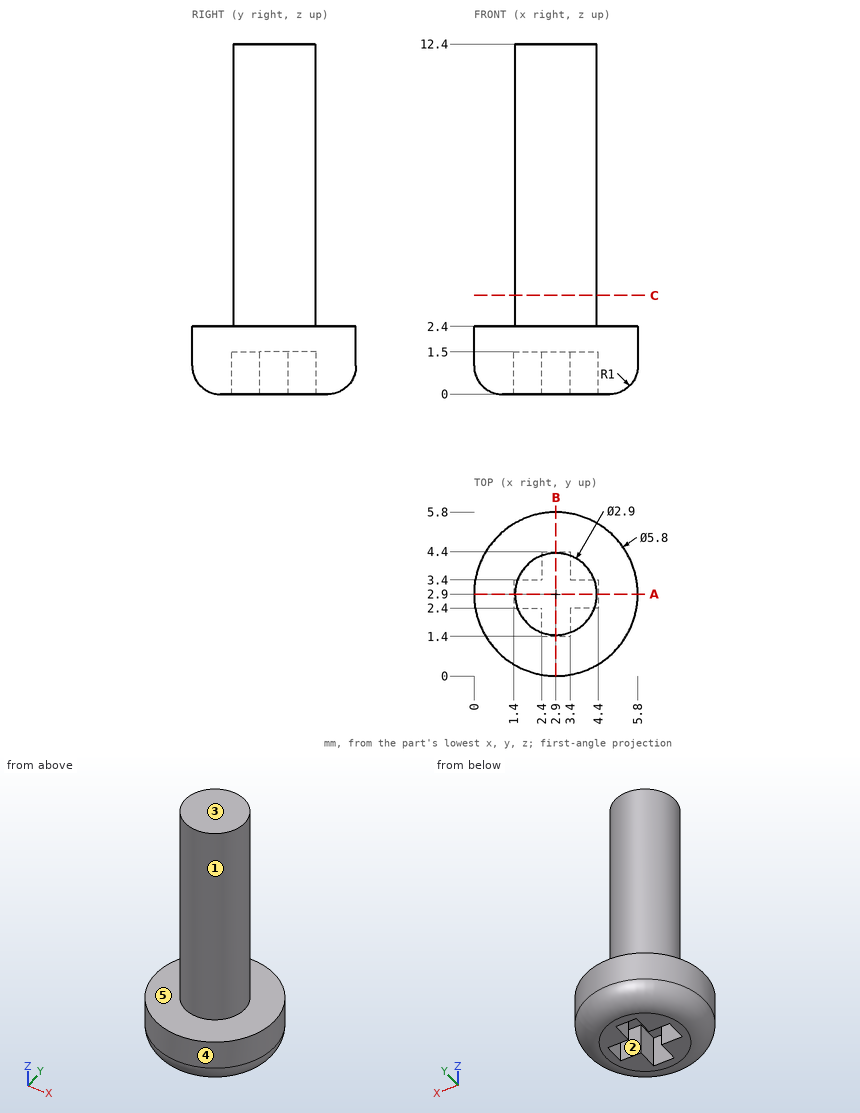
Geometry check sheet. Reference: drawing and pictorial views, mm from the part's lowest x, y, z. A direction names the side the tool comes from. Round coordinates to 2 decimals unless told otherwise and drop trailing zeros. Loops run counter-clockwise (first coordinate to the right, second up) from the corner with the lowest first, then second, coordinate; pieces in that order, holes last. Notation, with made-up numbers: (-30.75, -7.75) - (-2.75, -7.75) arc R8 cw to (-2.75, 1.25) - close; hole circle Ø2 at (-11.5, 0). An arc over 180 degrees is marked (long way). Answer in a Markdown table with one row per item. Add a question column.
Q1. Release check for a two-part mould opening along Y. For the marked faces 1, 2 and 3 record: pulls with the +Y half, pulls with the -Y half, needs draft (parallel to the pull), parting line crosses it, or undercut.
Q2. Section check A-A on y = 2.9. Enter the section's corners in (x, z).
Q3. Gauge pin test, flat ends, axial feed: pin 1 (0.5 mm diameter, centred on x = 2, z = 0.5, fed in from +Y); pin 2 (0.8 mm diameter, centred on x = 4, z = 1, fed in from -Y); pin 3 (0.8 mm diameter, centred on y = 4, z = 0.5, fed in from +X); pin 4 (1 mm diameter, centred on x = 5, z = 10, fed in from -Y). Record the tip position at first contact, or that the pin passes through.
Q4. Section check C-C on z = 3.5. Enter the section's corners in (x, y).
Q5. Material ranges on line 1 (Z direction, x = 2.65, y = 2.65); line 2 (X direction, y = 2.8, z = 2.5); line 3 (Z direction, x = 1.1, y = 3.2), recorded low to high.
Q6. Tool access check on the marked faces 4 and 5. Record the directions out of +Z, -Z, +X, -X, +Y, -Y that give a thin tool (end or side, any length) a straight path to the whole face; none if there is none.
Found:
| question | item | result |
|---|---|---|
| 1 | face 1 | parting line crosses it |
| 1 | face 2 | undercut |
| 1 | face 3 | needs draft |
| 2 | outline | (0, 1) arc R1 ccw to (1, 0) - (1.4, 0) - (1.4, 1.5) - (4.4, 1.5) - (4.4, 0) - (4.8, 0) arc R1 ccw to (5.8, 1) - (5.8, 2.4) - (4.35, 2.4) - (4.35, 12.4) - (1.45, 12.4) - (1.45, 2.4) - (0, 2.4) - close |
| 3 | pin 1 | stops at y = 5.65 |
| 3 | pin 2 | stops at y = 0.09 |
| 3 | pin 3 | stops at x = 5.66 |
| 3 | pin 4 | passes through |
| 4 | outline | circle Ø2.9 at (2.9, 2.9) |
| 5 | line 1 | z = 1.5 to 12.4 |
| 5 | line 2 | x = 1.45 to 4.35 |
| 5 | line 3 | z = 0 to 2.4 |
| 6 | face 4 | +Z, -Z |
| 6 | face 5 | +Z |
